The listing builds one solid part. Answer for the finished solid, in the listing's coordinates (mm). Face numbers are marked on the shaded views. A direction names the side the tool comes from. Coordinates: 2 decimals unless noted, no trailing zeros. Loops run counter-clockwise (first coordinate to the right, second up) from the corner with the lowest first, then second, coordinate; pieces in that order, holes last. Notation, with made-up numbers: (-13, -20.75) - (29, -20.75) arc R22 cw to (29, 7.25) - close; hole circle Ø9 at (32.5, 80.25). An arc over 180 degrees is marked (long way). Write each question's results on one line, items separated by ' | '. Start each with the question number.
(1) For the marked faces 1 and 2, determine the directions among +Z, -Z, +X, -X, +Y, -Y from which every point of the face is accessible in a straight line to the end or side of a thin tool.
(2) Find section A-A on x = 0.85. Determine the outline of the cut face in (y, z), then the cut area to 3 significant figures.
(3) Consider line 1 (X direction, y = -1.25, z = -2.25); line 2 (Z direction, x = 1, y = 0); line 3 (Z direction, x = 0.7, y = 0.5). Determine where each line is inside the solid, lowest interval first. Write a range as from..to.
(4) Determine the mould class of the marked faces 3, 4 and 5 for opening direction Z: released by +Z, released by -Z, zero draft, split by the parting line, or undercut.
(5) Given pin 1 Ø1.5 at (x, z) = (2.5, -0.5) entering from +Y; pin 2 Ø1.5 at (x, z) = (0, -1) entering from -Y; pin 3 Ø1.5 at (x, z) = (2.5, -2) entering from -Y, each flat-ended and moving along its own axis, determine where each tip first touches the part or whether it passes through.
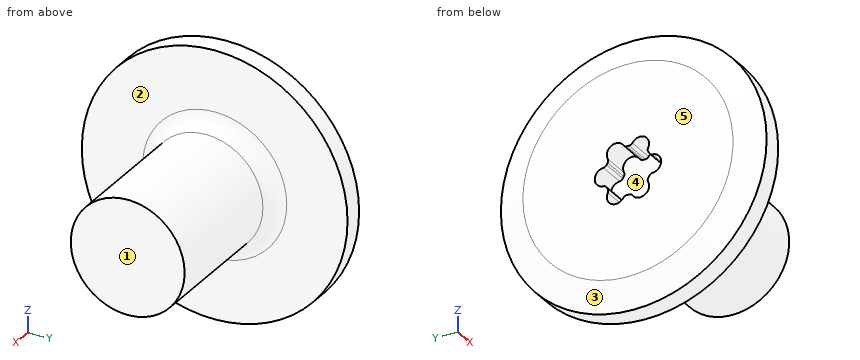
Autodesk Inventor part; units mm, degrees
ref_plane "YZ Plane" through (0, 0, 0) normal (1, 0, 0) x (0, 1, 0)
ref_plane "XZ Plane" through (0, 0, 0) normal (0, 1, 0) x (-1, 0, 0)
ref_plane "XY Plane" through (0, 0, 0) normal (0, 0, 1) x (1, 0, 0)
sketch "Sketch_1" plane through (0, 0, 0) normal (0, 0, 1) x (1, 0, 0)
  line L0 (6, 0) -> (0, 0)
  line L1 (-0.8, 0) -> (-0.8, 2.7673)
  line L2 (-0.8, 2.7673) -> (-0.5333, 3.5)
  line L3 (-0.5333, 3.5) -> (0, 3.5)
  line L4 (0, 3.5) -> (0, 1.9)
  arc A0 (0, 1.9) -> (0.4, 1.5) centre (0.4, 1.9) ccw
  line L5 (0.4, 1.5) -> (6, 1.5)
  line L6 (6, 1.5) -> (6, 0)
  line L7 (6, 0) -> (-0.8, 0)
  line L8 (0, 0) -> (-0.8, 0)
  dimension "d6" = 6
revolve "Revolution1" add sketch "Sketch_1" angle 360 about axis through (6, 0, 0) along (1, 0, 0)
thread "Thread1"
sketch "Sketch_5" plane through (-0.05, 0, 0) normal (1, 0, 0) x (0, 0, -1)
  arc A0 (-0.6801, -0.1159) -> (-0.4404, -0.531) centre (-0.5499, -0.3175) ccw
  arc A1 (-0.341, -0.5357) -> (-0.4404, -0.531) centre (-0.3947, -0.62) ccw
  arc A2 (-0.341, -0.5357) -> (-0.2934, -0.5632) centre (0, 0) ccw
  arc A3 (-0.2397, -0.6469) -> (-0.2934, -0.5632) centre (-0.3396, -0.6519) ccw
  arc A4 (-0.2397, -0.6469) -> (0.2397, -0.6469) centre (0, -0.635) ccw
  arc A5 (0.2934, -0.5632) -> (0.2397, -0.6469) centre (0.3396, -0.6519) ccw
  arc A6 (0.2934, -0.5632) -> (0.341, -0.5357) centre (0, 0) ccw
  arc A7 (0.4404, -0.531) -> (0.341, -0.5357) centre (0.3947, -0.62) ccw
  arc A8 (0.4404, -0.531) -> (0.6801, -0.1159) centre (0.5499, -0.3175) ccw
  arc A9 (0.6344, -0.0275) -> (0.6801, -0.1159) centre (0.7343, -0.0318) ccw
  arc A10 (0.6344, -0.0275) -> (0.6344, 0.0275) centre (0, 0) ccw
  arc A11 (0.6801, 0.1159) -> (0.6344, 0.0275) centre (0.7343, 0.0318) ccw
  arc A12 (0.6801, 0.1159) -> (0.4404, 0.531) centre (0.5499, 0.3175) ccw
  arc A13 (0.341, 0.5357) -> (0.4404, 0.531) centre (0.3947, 0.62) ccw
  arc A14 (0.341, 0.5357) -> (0.2934, 0.5632) centre (0, 0) ccw
  arc A15 (0.2397, 0.6469) -> (0.2934, 0.5632) centre (0.3396, 0.6519) ccw
  arc A16 (0.2397, 0.6469) -> (-0.2397, 0.6469) centre (0, 0.635) ccw
  arc A17 (-0.2934, 0.5632) -> (-0.2397, 0.6469) centre (-0.3396, 0.6519) ccw
  arc A18 (-0.2934, 0.5632) -> (-0.341, 0.5357) centre (0, 0) ccw
  arc A19 (-0.4404, 0.531) -> (-0.341, 0.5357) centre (-0.3947, 0.62) ccw
  arc A20 (-0.4404, 0.531) -> (-0.6801, 0.1159) centre (-0.5499, 0.3175) ccw
  arc A21 (-0.6344, 0.0275) -> (-0.6801, 0.1159) centre (-0.7343, 0.0318) ccw
  arc A22 (-0.6344, 0.0275) -> (-0.6344, -0.0275) centre (0, 0) ccw
  arc A23 (-0.6801, -0.1159) -> (-0.6344, -0.0275) centre (-0.7343, -0.0318) ccw
extrude "Extrusion1" cut sketch "Sketch_5" against normal blind 0.75
sketch "Sketch_2" plane through (0, 0, 0) normal (0, 0, 1) x (1, 0, 0)
  line L0 (0.4552, 0) -> (0, 0)
  line L1 (-0.05, 0) -> (-0.05, 0.875)
  line L2 (-0.05, 0.875) -> (0.4552, 0)
  line L3 (0.4552, 0) -> (-0.05, 0)
revolve "Revolution2" cut sketch "Sketch_2" angle 360 about axis through (0.4552, 0, 0) along (1, 0, 0)
sketch "スケッチ4" plane through (6, 0, 0) normal (1, 0, 0) x (0, 0, -1)
  circle A0 centre (0, 0) radius 1.5
extrude "押し出し2" cut sketch "スケッチ4" against normal blind 2
properties part number "超極低頭ネジL4" material "ステンレス鋼"
Values:
1) face 1: +Z, -Z, +X, +Y, -Y | face 2: +X
2) outline: circle Ø3 at (0, 0) | area: 7.07 mm²
3) line 1: x = -0.8..0 | line 2: z = -1.5..1.5 | line 3: z = -1.41..1.41
4) face 3: split by the parting line | face 4: undercut | face 5: zero draft
5) pin 1: stops at y = 1.5 | pin 2: stops at y = -3.49 | pin 3: stops at y = -0.83
